Check sheet for the modelled part. Datum: model origin and axes. Units: mm. A direction names the side the tool comes from. Coordinates: 2 decimals unless noted, no trailing zeros. Loops run counter-clockwise (first coordinate to the right, second up) from the corner with the lowest first, then second, coordinate; pieces in that order, holes last.
from build123d import *

# Parameters (mm, degrees)
F0_W     = 260.01095
F0_H     = 108.525954
F1_DEPTH = 25.4
F2_R     = 15.61088
F2_R_2   = 21.151668
F2_R_3   = 18.900746
F3_DEPTH = 25.4


with BuildPart() as f1:
    # F0 (on Top) → F1 (new body)
    with BuildSketch(Plane.XY):
        with Locations((5.983893, -12.487542)):
            Rectangle(F0_W, F0_H)
    extrude(amount=F1_DEPTH)

    # F2 (on face) → F3 (join)
    with BuildSketch(Plane.XY.offset(25.4)):
        with Locations((-68.63334, -13.820079)):
            Circle(F2_R)
        with Locations((8.536131, -15.846584)):
            Circle(F2_R_2)
        with Locations((83.193891, -15.645826)):
            Circle(F2_R_3)
    extrude(amount=F3_DEPTH)


solid = f1.part
(1) Section check A-A, the plane x = 7. Enter the section's corners in (y, z).
(2) Section check B-B, the plane y = -10. Enter the section's corners in (x, z), plus the area to 3 significant figures.
(3) Section check D-D, the plane x = -71. Enter the section's corners in (y, z).
(4) Gauge pin test, flat ends, axial feed: P1, Ø12, axis at x = -24.5, y = -4, coming from the +Z side; P2, Ø1, axis at x = -98, y = -51.5, coming from the -Z side; P3, Ø12, axis at x = 10.5, z = 34.5, coming from the -Y side; P4, Ø12, axis at y = -11, z = 40, coming from the -X side. Record the tip position at first contact, or that the pin passes through.
(5) Draft check along X on faces 3 (the face through (8, -16, 50.8)), 4 (the face through (135.989, -13, 13)), 5 (the face through (100.653, -22.885, 37.922)). Enter one of: pulls with the +X half, pulls with the -X half, needs draft (parallel to the pull), parting line crosses it, or undercut.
(6) Section check C-C, the plane z = 40.5. Enter the section's corners in (x, y).
(7) Scan lines: line 1 along X through (y, z) = (-27.5, 47); line 2 along Z through (x, y) = (51, -8); line 3 along X through (y, z) = (-8, 39). Record each from-to range of solid material in increasing order.
(8) Set-up check for faces 1 (the face through (-54.213, -19.799, 37.922)), 2 (the face through (83, -15, 50.8)): record each of +Z, -Z, +X, -X, +Y, -Y from which the full face is reachable in a straight line by a thin tool's end or side.
Determined:
1. outline: (-66.75, 0) - (41.78, 0) - (41.78, 25.4) - (5.25, 25.4) - (5.25, 50.8) - (-36.94, 50.8) - (-36.94, 25.4) - (-66.75, 25.4) - close
2. outline: (-124.02, 0) - (135.99, 0) - (135.99, 25.4) - (101.23, 25.4) - (101.23, 50.8) - (65.16, 50.8) - (65.16, 25.4) - (28.86, 25.4) - (28.86, 50.8) - (-11.79, 50.8) - (-11.79, 25.4) - (-53.5, 25.4) - (-53.5, 50.8) - (-83.77, 50.8) - (-83.77, 25.4) - (-124.02, 25.4) - close
2. area: 9,320 mm2
3. outline: (-66.75, 0) - (41.78, 0) - (41.78, 25.4) - (1.61, 25.4) - (1.61, 50.8) - (-29.25, 50.8) - (-29.25, 25.4) - (-66.75, 25.4) - close
4. P1: stops at z = 25.4
4. P2: stops at z = 0
4. P3: stops at y = -37
4. P4: stops at x = -84.24
5. face 3: needs draft
5. face 4: pulls with the +X half
5. face 5: undercut
6. outline: circle Ø31.22 at (-68.63, -13.82); circle Ø42.3 at (8.54, -15.85); circle Ø37.8 at (83.19, -15.65)
7. line 1: x = -76.15 to -61.11, -9.12 to 26.19, 68.47 to 97.92
7. line 2: z = 0 to 25.4
7. line 3: x = -83.12 to -54.15, -11.11 to 28.18, 65.91 to 100.48
8. face 1: +Z
8. face 2: +Z, +X, -X, +Y, -Y
